from build123d import *

# Parameters (mm, degrees)
F0_W     = 50
F0_H     = 50
F1_DEPTH = 450
F3_DEPTH = 50.001
F4_R     = 9
F5_DEPTH = 25


with BuildPart() as f1:
    # F0 (on Front) → F1 (new body)
    with BuildSketch(Plane.XZ):
        Rectangle(F0_W, F0_H)
    extrude(amount=F1_DEPTH)

    # F2 (on face) → F3 (cut, through all)
    with BuildSketch(Plane.YZ.offset(25)):
        Polygon((-400, 25), (-450, 25), (-450, -25), align=None)
    extrude(amount=-F3_DEPTH, mode=Mode.SUBTRACT)

    # F4 (on face) → F5 (cut)
    with BuildSketch(Plane.XY.offset(25)):
        with Locations((0, -25)):
            Circle(F4_R)
    extrude(amount=-F5_DEPTH, mode=Mode.SUBTRACT)


solid = f1.part
The model under review builds one solid part; all positions refer to its coordinate system, in mm. A direction names the side the tool comes from. Coordinates: 2 decimals unless noted, no trailing zeros. Loops run counter-clockwise (first coordinate to the right, second up) from the corner with the lowest first, then second, coordinate; pieces in that order, holes last.
(1) Consider section B-B, the plane x = 0. Give the boundary of the cut face in (y, z), plus the area to 3 significant figures.
Determined:
outline: (-450, -25) - (0, -25) - (0, 25) - (-16, 25) - (-16, 0) - (-34, 0) - (-34, 25) - (-400, 25) - close
area: 20,800 mm2
(2) Consider section A-A, the plane z = 11. Give the boundary of the cut face in (x, y), plus the area to 3 significant figures.
Determined:
outline: (-25, -414) - (25, -414) - (25, 0) - (-25, 0) - close; hole circle Ø18 at (0, -25)
area: 20,400 mm2
(3) Consider section C-C, the plane y = -25. Give the boundary of the cut face in (x, z), plus the area to 3 significant figures.
Determined:
outline: (-25, -25) - (25, -25) - (25, 25) - (9, 25) - (9, 0) - (-9, 0) - (-9, 25) - (-25, 25) - close
area: 2,050 mm2
(4) Insertion check: P1, Ø3, axis at x = -6.5, z = 2, coming from the -Y side; P2, Ø14.5, axis at x = 2, y = -25.5, coming from the +Z side; P3, Ø3, axis at x = 3.5, z = 0.5, coming from the -Y side. Each pin has a flat end and moves straight along its axis. Give the tip position at first contact, or say it passes through.
Determined:
P1: stops at y = -424.5
P2: stops at z = 25
P3: stops at y = -426
(5) Consider section D-D, the plane z = -17. Give the boundary of the cut face in (x, y).
Determined:
outline: (-25, -442) - (25, -442) - (25, 0) - (-25, 0) - close
(6) Tool access review of faces 4 (the flat face through (0, -197, 25)), 5 (the flat face through (0, -25, 0)): name each direction out of +Z, -Z, +X, -X, +Y, -Y from which nothing blocks a thin tool from reaching the whole face with its end or side.
Determined:
face 4: +Z, +X, -X, +Y, -Y
face 5: +Z
(7) Draft analysis for pull direction Y (two halves, no side actions). For faces 1 (the flat face through (0, 0, 0)), 2 (the cylindrical face through (-1.172, -16.077, 12.675)), 3 (the flat face through (0, -425, 0)), state which applies: +Y half, -Y half, draft (parallel to the pull), parting line (faces both ways), or undercut.
Determined:
face 1: +Y half
face 2: undercut
face 3: -Y half
(8) Wall thickness on L1, parallel to Y at x = 0, z = 12.25; L2, parallel to Y at x = 0, z = 17; L3, parallel to Y at x = 12, z = 15.5: over which ranges is each line inside the solid? List them lowest first.
Determined:
L1: y = -412.75 to -34, -16 to 0
L2: y = -408 to -34, -16 to 0
L3: y = -409.5 to 0
